```python
from build123d import *

# Parameters (mm, degrees)
EXTRUDE_THIN1_DEPTH = 82.55
SKETCH2_R           = 2.413
EXTRUDE2_DEPTH      = 87.794442541
LPATTERN1_COUNT     = 13
LPATTERN1_PITCH     = 12.7
FILLET1_R           = 6.35
SKETCH3_R           = 2.413
EXTRUDE3_DEPTH      = 87.294607595
LPATTERN2_COUNT     = 13
LPATTERN2_PITCH     = 76.2
EXTRUDE4_DEPTH      = 87.294607595


with BuildPart() as part:
    # Sketch1 → Extrude-Thin1 (new, symmetric)
    with BuildSketch(Plane(origin=(0, 0, 0), x_dir=(0, 0, -1), z_dir=(1, 0, 0))):
        with BuildLine():
            Line((0, 0), (15.494, 0))
            ThreePointArc((15.494, 0), (17.110446102, 0.669553898), (17.78, 2.286))
            Line((17.78, 2.286), (17.78, 17.78))
            Line((17.78, 17.78), (20.066, 17.78))
            Line((20.066, 17.78), (20.066, 2.286))
            ThreePointArc((20.066, 2.286), (18.726892204, -0.946892204), (15.494, -2.286))
            Line((15.494, -2.286), (0, -2.286))
            Line((0, -2.286), (0, 0))
        make_face()
    extrude(amount=EXTRUDE_THIN1_DEPTH, both=True)

    # Sketch2 → Extrude2 (cut, through all)
    with BuildSketch(Plane(origin=(0, 0, 0), x_dir=(-1, 0, 0), z_dir=(0, 1, 0))):
        with Locations(Location((76.2, -6.35, 0), (0, 0, 90))):
            Circle(SKETCH2_R)
    extrude2 = extrude(amount=-EXTRUDE2_DEPTH, mode=Mode.SUBTRACT)

    # LPattern1: Extrude2 ×13
    with Locations(*[(i * LPATTERN1_PITCH, 0, 0) for i in range(1, LPATTERN1_COUNT)]):
        add(extrude2, mode=Mode.SUBTRACT)

    # Fillet1
    fillet1_edges = [part.edges().sort_by_distance(p)[0] for p in [
        (82.55, -1.143, 0),
        (-82.55, -1.143, 0),
        (82.55, 17.78, -18.923),
        (-82.55, 17.78, -18.923),
    ]]
    fillet(fillet1_edges, radius=FILLET1_R)

    # Sketch3 → Extrude3 (cut, through all)
    with BuildSketch(Plane.XY.offset(-17.78)):
        with Locations((-76.2, 11.43)):
            Circle(SKETCH3_R)
    extrude3 = extrude(amount=-EXTRUDE3_DEPTH, mode=Mode.SUBTRACT)

    # LPattern2: Extrude3 ×13
    with Locations(*[(i * LPATTERN2_PITCH, 0, 0) for i in range(1, LPATTERN2_COUNT)]):
        add(extrude3, mode=Mode.SUBTRACT)

    # Sketch4 → Extrude4 (cut, through all)
    with BuildSketch(Plane.XY.offset(-17.78)):
        with BuildLine():
            Line((-63.5, 13.843), (-12.7, 13.843))
            ThreePointArc((-12.7, 13.843), (-10.287, 11.43), (-12.7, 9.017))
            Line((-12.7, 9.017), (-63.5, 9.017))
            ThreePointArc((-63.5, 9.017), (-65.913, 11.43), (-63.5, 13.843))
        make_face()
        with BuildLine():
            Line((63.5, 13.843), (12.7, 13.843))
            ThreePointArc((12.7, 13.843), (10.287, 11.43), (12.7, 9.017))
            Line((12.7, 9.017), (63.5, 9.017))
            ThreePointArc((63.5, 9.017), (65.913, 11.43), (63.5, 13.843))
        make_face()
    extrude(amount=-EXTRUDE4_DEPTH, mode=Mode.SUBTRACT)


solid = part.part
```
Geometry check sheet. Reference: the model listing, model coordinates, mm. A direction names the side the tool comes from. Coordinates: 2 decimals unless noted, no trailing zeros. Order: outer loops, then holes, each group sorted by start corner. A loop starts at its lowest first (then second) coordinate and runs counter-clockwise, first axis right, second up. Notation, with made-up numbers: (17, 85.5) - (22, 85.5) arc R31 cw to (22, 114.5) - close; hole circle Ø3 at (-4, 82.25). An arc over 180 degrees is marked (long way). Answer in a Markdown table with one row per item. Add a question column.
1. Section check D-D (y = 7.5). Enter the section's corners in (x, z), plus the area to 3 significant figures.
2. Material ranges on L1, parallel to Y at x = 22, z = -11.75; L2, parallel to Z at x = 0, y = -1.05; L3, parallel to Z at x = -42, y = 3.5, recorded low to high. Write a range as [from, to].
3. Section check B-B (x = 19.5). Enter the section's corners in (y, z), plus the area to 3 significant figures.
4. Draft check along X on faces 1 (the face through (73.79, 11.54, -18.91)), 2 (the face through (80.74, 15.87, -18.94)), 3 (the face through (-82.55, 2, -18)). Enter one of: +X half, -X half, draft (parallel to the pull), parting line (faces both ways), or undercut.
5. Access from +Z, -Z, +X, -X, +Y, -Y to the whole of each face (thin tool, end or side, straight path). Record for faces 4 (the face through (80.64, -1.13, -1.81)), 5 (the face through (1, 8, -17.78)).
6. Gauge pin test, flat ends, axial feed: pin 1 Ø3 at (x, y) = (-41, 15) entering from +Z; pin 2 Ø3 at (x, z) = (-25.4, -6.35) entering from -Y; pin 3 Ø1.8 at (x, z) = (-45.5, -18.5) entering from -Y; pin 4 Ø7.5 at (x, z) = (38.1, -6.35) entering from +Y. Record the tip position at first contact, or that the pin passes through.
7. Section check C-C (x = 69). Enter the section's corners in (y, z), plus the area to 3 significant figures.
8. Section check A-A (x = 50.8). Enter the section's corners in (y, z).
Data:
| question | item | result |
|---|---|---|
| 1 | outline | (-82.55, -20.07) - (82.55, -20.07) - (82.55, -17.78) - (-82.55, -17.78) - close |
| 1 | area | 377 mm² |
| 2 | L1 | y = [-2.29, 0] |
| 2 | L2 | z = [-18.62, -8.76], [-3.94, 0] |
| 2 | L3 | z = [-20.07, -17.78] |
| 3 | outline | (-2.29, -15.49) arc R4.57 ccw to (2.29, -20.07) - (9.02, -20.07) - (9.02, -17.78) - (2.29, -17.78) arc R2.29 cw to (0, -15.49) - (0, 0) - (-2.29, 0) - close; (13.84, -20.07) - (17.78, -20.07) - (17.78, -17.78) - (13.84, -17.78) - close |
| 3 | area | 72.1 mm² |
| 4 | face 1 | undercut |
| 4 | face 2 | +X half |
| 4 | face 3 | -X half |
| 5 | face 4 | +Z, +X, +Y, -Y |
| 5 | face 5 | +Z, +X, -X, +Y |
| 6 | pin 1 | stops at z = -17.78 |
| 6 | pin 2 | passes through |
| 6 | pin 3 | stops at y = -1.77 |
| 6 | pin 4 | stops at y = 0 |
| 7 | outline | (-2.29, -15.49) arc R4.57 ccw to (2.29, -20.07) - (17.78, -20.07) - (17.78, -17.78) - (2.29, -17.78) arc R2.29 cw to (0, -15.49) - (0, 0) - (-2.29, 0) - close |
| 7 | area | 83.2 mm² |
| 8 | outline | (-2.29, -15.49) arc R4.57 ccw to (2.29, -20.07) - (9.02, -20.07) - (9.02, -17.78) - (2.29, -17.78) arc R2.29 cw to (0, -15.49) - (0, -8.76) - (-2.29, -8.76) - close; (-2.29, -3.94) - (0, -3.94) - (0, 0) - (-2.29, 0) - close; (13.84, -20.07) - (17.78, -20.07) - (17.78, -17.78) - (13.84, -17.78) - close |
